from build123d import *

# Parameters (mm, degrees)
F0_W          = 125
F0_H          = 40
F1_DEPTH      = 10
F3_DEPTH      = 50
F4_W          = 20
F4_H          = 10
F5_DEPTH      = 40
F5_DEPTH_BACK = 25
F7_DEPTH      = 40
F8_W          = 5
F8_H          = 15
F9_DEPTH      = 30


with BuildPart() as f1:
    # F0 (on Front) → F1 (new body)
    with BuildSketch(Plane.XZ):
        Rectangle(F0_W, F0_H)
    extrude(amount=F1_DEPTH)

    # F2 (on face) → F3 (join)
    with BuildSketch(Plane(origin=(-62.5, 0, 0), x_dir=(0, -1, 0), z_dir=(-1, 0, 0))):
        Polygon((-20, -20), (0, -20), (0, 0), (-30, 0), (-30, -5), (-20, -5), align=None)
        Polygon((-30, 0), (0, 0), (0, 20), (-20, 20), (-20, 5), (-30, 5), align=None)
    extrude(amount=-F3_DEPTH)

    # F4 (on face) → F5 (cut, two sides)
    with BuildSketch(Plane.XY.offset(20)) as f5_sk:
        with Locations((-37.5, 5)):
            Rectangle(F4_W, F4_H)
    extrude(amount=-F5_DEPTH, mode=Mode.SUBTRACT)
    extrude(f5_sk.sketch, amount=-F5_DEPTH_BACK, mode=Mode.SUBTRACT)

    # F6 (on face) → F7 (join)
    with BuildSketch(Plane.XY.offset(20)):
        Polygon((101.471143, 22.5), (62.5, 0), (62.5, -10), (106.471143, 13.839746), align=None)
    extrude(amount=-F7_DEPTH)

    # F8 (on face) → F9 (cut)
    with BuildSketch(Plane(origin=(85.846143, 49.563294, 0), x_dir=(-0.5, 0.866025, 0), z_dir=(0.866025, 0.5, 0))):
        with Locations((-36.25, -12.5)):
            Rectangle(F8_W, F8_H)
        with Locations((-36.25, 12.5)):
            Rectangle(F8_W, F8_H)
    extrude(amount=-F9_DEPTH, mode=Mode.SUBTRACT)


solid = f1.part
Could you check a few things on this model? Use its own coordinates, in mm. A direction names the side the tool comes from. Give positions to 0.01 mm unless a question says otherwise; leave off trailing zeros. Order: outer loops, then holes, each group sorted by start corner. A loop starts at its lowest first (then second) coordinate and runs counter-clockwise, first axis right, second up.
Item 1: If we section it at B-B, the plane z = -8.5: Write out the boundary of the cut face in (x, y).
Item 2: If we section it at D-D, the plane y = 3.5: Write out the boundary of the cut face in (x, z), plus the area to 3 significant figures.
Item 3: For faces 4 (the face through (92.41, 8.61, -12.6)), 5 (the face through (24, 0, 0)), 6 (the face through (-38, 20, 13)), 7 (the face through (78.008, 3.14, 12.605)), 8 (the face through (-47.5, 5, 0)), which set-ups out of +Z, -Z, +X, -X, +Y, -Y let a thin tool reach every point of the face, with its end or its side?
Item 4: I need wall thicknesses on line 1 (X direction, y = 9, z = -11.5); line 2 (Y direction, x = -34, z = 2.5); line 3 (Y direction, x = -38.5, z = 14.5). Which ranges of each line are inside material? Lowest first, please.
Item 5: If we section it at C-C, the plane x = -21.5: Write out the boundary of the cut face in (y, z).
Item 6: If we section it at A-A, the plane x = -39.5: Write out the boundary of the cut face in (y, z).
Item 7: I'm going to push flat-ended pins straight in: pin 1 (7.5 mm diameter, centred on x = -27.5, z = -10, fed in from +Y); pin 2 (3 mm diameter, centred on x = -50, y = 23, fed in from -Z); pin 3 (8 mm diameter, centred on y = 3, z = 3, fed in from +X). Where does each tip first touch, or does it pass through?
Item 8: If we mould it in two halves opening along X, with no side actions, what happens to faces 1 (the face through (104.006, 18.109, 0.28)), 2 (the face through (91, 11, 5)), 3 (the face through (-1, -10, 0))? For each: pulls with the +X half, pulls with the -X half, needs draft (parallel to the pull), parting line crosses it, or undercut.
Values:
1. outline: (-62.5, -10) - (62.5, -10) - (106.47, 13.84) - (105.22, 16) - (79.24, 1) - (76.74, 5.33) - (102.72, 20.33) - (101.47, 22.5) - (62.5, 0) - (-12.5, 0) - (-12.5, 20) - (-62.5, 20) - close; hole (-47.5, 0) - (-27.5, 0) - (-27.5, 10) - (-47.5, 10) - close
2. outline: (-62.5, -20) - (-47.5, -20) - (-47.5, 20) - (-62.5, 20) - close; (-27.5, -20) - (-12.5, -20) - (-12.5, 20) - (-27.5, 20) - close; (68.56, -20) - (77.8, -20) - (77.8, -5) - (83.56, -5) - (83.56, -20) - (87.4, -20) - (87.4, 20) - (83.56, 20) - (83.56, 5) - (77.8, 5) - (77.8, 20) - (68.56, 20) - close
2. area: 1,780 mm2
3. face 4: -Z
3. face 5: +Z, -Z, +Y
3. face 6: +Z, -X, +Y
3. face 7: +Z
3. face 8: +Z, -Z
4. line 1: x = -62.5 to -47.5, -27.5 to -12.5, 78.09 to 83.09, 93.09 to 97.54
4. line 2: y = -10 to 0, 10 to 30
4. line 3: y = -10 to 0, 10 to 20
5. outline: (-10, -20) - (20, -20) - (20, -5) - (30, -5) - (30, 5) - (20, 5) - (20, 20) - (-10, 20) - close
6. outline: (-10, -20) - (0, -20) - (0, 20) - (-10, 20) - close; (10, -20) - (20, -20) - (20, -5) - (30, -5) - (30, 5) - (20, 5) - (20, 20) - (10, 20) - close
7. pin 1: stops at y = 20
7. pin 2: stops at z = -5
7. pin 3: stops at x = 93.86
8. face 1: pulls with the +X half
8. face 2: undercut
8. face 3: needs draft
